Check sheet for the modelled part. Datum: model origin and axes. Units: mm. Coordinates: 2 decimals unless noted, no trailing zeros. Loops run counter-clockwise (first coordinate to the right, second up) from the corner with the lowest first, then second, coordinate; pieces in that order, holes last. Notation, with made-up numbers: (-16, 21) -> (-1, 21) arc R31 ccw to (-1, 53) -> close; hole circle Ø8 at (18, -36.5). An arc over 180 degrees is marked (long way). Use one line per item in the form item = value.
from build123d import *

# Parameters (mm, degrees)
F0_R     = 11
F1_DEPTH = 3


with BuildPart() as f1:
    # F0 (on Top) → F1 (new body)
    with BuildSketch(Plane.XY):
        with BuildLine():
            add(Edge.make_bspline(
                [(5.0692520794, 26.9407597389), (1.3719432198, 30.1629827921), (-1.3719432198, 30.1629827921), (-5.0692520794, 26.9407597389)],
                knots=[0.8898242879, 0.8898242879, 0.8898242879, 0.8898242879, 1, 1, 1, 1], degree=3))
            ThreePointArc((5.0692520794, 26.9407597389), (0, 56.0582199693), (-5.0692520794, 26.9407597389))
        make_face()
        with Locations((0, 41.0582199693)):
            Circle(F0_R, mode=Mode.SUBTRACT)
        with BuildLine():
            add(Edge.make_bspline(
                [(25.8660083708, -9.0802787905), (23.9582735086, 0.6684610246), (12.5580409831, 20.414242977), (5.0692520794, 26.9407597389)],
                knots=[0.6666666667, 0.6666666667, 0.6666666667, 0.6666666667, 0.8898242879, 0.8898242879, 0.8898242879, 0.8898242879], degree=3))
            add(Edge.make_bspline(
                [(5.0692520794, 26.9407597389), (1.3719432198, 30.1629827921), (-1.3719432198, 30.1629827921), (-5.0692520794, 26.9407597389)],
                knots=[0.8898242879, 0.8898242879, 0.8898242879, 0.8898242879, 1, 1, 1, 1], degree=3))
            add(Edge.make_bspline(
                [(-5.0692520794, 26.9407597389), (-12.5580409831, 20.414242977), (-23.9582735086, 0.6684610246), (-25.8660083708, -9.0802787905)],
                knots=[0, 0, 0, 0, 0.2231576212, 0.2231576212, 0.2231576212, 0.2231576212], degree=3))
            add(Edge.make_bspline(
                [(-25.8660083708, -9.0802787905), (-26.8078809618, -13.8933537152), (-25.435937742, -16.2696290769), (-20.7967562915, -17.8604809484)],
                knots=[0.2231576212, 0.2231576212, 0.2231576212, 0.2231576212, 0.3333333333, 0.3333333333, 0.3333333333, 0.3333333333], degree=3))
            add(Edge.make_bspline(
                [(-20.7967562915, -17.8604809484), (-11.4002325256, -21.0827040016), (11.4002325256, -21.0827040016), (20.7967562915, -17.8604809484)],
                knots=[0.3333333333, 0.3333333333, 0.3333333333, 0.3333333333, 0.5564909546, 0.5564909546, 0.5564909546, 0.5564909546], degree=3))
            add(Edge.make_bspline(
                [(20.7967562915, -17.8604809484), (25.435937742, -16.2696290769), (26.8078809618, -13.8933537152), (25.8660083708, -9.0802787905)],
                knots=[0.5564909546, 0.5564909546, 0.5564909546, 0.5564909546, 0.6666666667, 0.6666666667, 0.6666666667, 0.6666666667], degree=3))
        make_face()
        Circle(F0_R, mode=Mode.SUBTRACT)
        with BuildLine():
            ThreePointArc((20.7967562915, -17.8604809484), (48.5478425843, -28.0291099846), (25.8660083708, -9.0802787905))
            add(Edge.make_bspline(
                [(20.7967562915, -17.8604809484), (25.435937742, -16.2696290769), (26.8078809618, -13.8933537152), (25.8660083708, -9.0802787905)],
                knots=[0.5564909546, 0.5564909546, 0.5564909546, 0.5564909546, 0.6666666667, 0.6666666667, 0.6666666667, 0.6666666667], degree=3))
        make_face()
        with Locations((35.5574615276, -20.5291099846)):
            Circle(F0_R, mode=Mode.SUBTRACT)
        with BuildLine():
            add(Edge.make_bspline(
                [(-25.8660083708, -9.0802787905), (-26.8078809618, -13.8933537152), (-25.435937742, -16.2696290769), (-20.7967562915, -17.8604809484)],
                knots=[0.2231576212, 0.2231576212, 0.2231576212, 0.2231576212, 0.3333333333, 0.3333333333, 0.3333333333, 0.3333333333], degree=3))
            ThreePointArc((-25.8660083708, -9.0802787905), (-48.5478425843, -28.0291099846), (-20.7967562915, -17.8604809484))
        make_face()
        with Locations((-35.5574615276, -20.5291099846)):
            Circle(F0_R, mode=Mode.SUBTRACT)
    extrude(amount=F1_DEPTH)


solid = f1.part
(1) Section check C-C, the plane x = 0. Give the number of separate pieces and of enclosed holes in the cut face, plus the area to 3 significant figures.
Established:
separate_pieces = 3
enclosed_holes = 0
area = 97.0 mm²
(2) Mould release check, pull along Y, two halves, no side actions. Record for faces 1 (the flat face through (0, -13, 0)), 2 (the cylindrical face through (-36.989, -9.623, 1.479)): +Y half, -Y half, draft (parallel to the pull), parting line (faces both ways), or undercut.
Established:
face_1 = draft
face_2 = undercut
(3) Section check B-B, the plane y = -28.5. Record the boundary of the cut face in (x, z).
Established:
outline = (-48.26, 0) -> (-43.14, 0) -> (-43.14, 3) -> (-48.26, 3) -> close; (-27.98, 0) -> (-22.85, 0) -> (-22.85, 3) -> (-27.98, 3) -> close; (22.85, 0) -> (27.98, 0) -> (27.98, 3) -> (22.85, 3) -> close; (43.14, 0) -> (48.26, 0) -> (48.26, 3) -> (43.14, 3) -> close
(4) Go/stop test with a flat-tipped pin: P1, Ø1, axis at x = -18, y = -21, coming from the -Z side. Record where the tip stops, or that it passes through.
Established:
P1 = through
(5) Section check A-A, the plane y = 50.5. Record the boundary of the cut face in (x, z), plus the area to 3 significant figures.
Established:
outline = (-11.66, 0) -> (-5.64, 0) -> (-5.64, 3) -> (-11.66, 3) -> close; (5.64, 0) -> (11.66, 0) -> (11.66, 3) -> (5.64, 3) -> close
area = 36.1 mm²
(6) Scan lines: line 1 along Y through (x, z) = (0, 1.6); line 2 along Y through (x, z) = (-8.5, 0.2); line 3 along X through (y, z) = (-8, 0.8). Record each from-to range of solid material in increasing order.
Established:
line_1 = -20.28 to -11, 11 to 30.06, 52.06 to 56.06
line_2 = -19.97 to -6.98, 6.98 to 23.38, 28.7 to 34.08, 48.04 to 53.42
line_3 = -43.8 to -27.31, -25.63 to -7.55, 7.55 to 25.63, 27.31 to 43.8
